Model file for the job. Use its own axes, mm. Give positions to 0.01 mm unless a question says otherwise; leave off trailing zeros. Write each loop counter-clockwise with the first axis right and the second up, starting at its lowest first coordinate (ties: lowest second). Pieces come first, ordered by that corner, then holes. Notation, with made-up numbers: (48, -32) - (77, -32) arc R25 cw to (77, 5) - close; hole circle Ø1 at (87.25, -9). An arc over 180 degrees is marked (long way). Use CSV: the item, a comma, the result in double quotes.
from build123d import *

# Parameters (mm, degrees)
BOSS_EXTRUDE1_DEPTH         = 3.175
FILLET1_R                   = 3.175
F_1_4_0_25_DIAMETER_HOLE1_D = 6.35


with BuildPart() as part:
    # Sketch1 → Boss-Extrude1 (new body)
    with BuildSketch(Plane(origin=(0, 0, 0), x_dir=(1, 0, 0), z_dir=(0, 1, 0))):
        Polygon((-634.164473684, 176.797368421), (413.585526316, 75.197368421), (413.585526316, -115.302631579), (-634.164473684, -115.302631579), align=None)
    extrude(amount=BOSS_EXTRUDE1_DEPTH)

    # Fillet1
    fillet1_edges = [part.edges().sort_by_distance(p)[0] for p in [
        (413.585526316, 1.5875, 115.302631579),
        (-634.164473684, 1.5875, 115.302631579),
        (-634.164473684, 1.5875, -176.797368421),
        (413.585526316, 1.5875, -75.197368421),
    ]]
    fillet(fillet1_edges, radius=FILLET1_R)

    # 1/4 (0.25) Diameter Hole1 (through all)
    with Locations(Plane(origin=(0, 3.175, 0), x_dir=(1, 0, 0), z_dir=(0, 1, 0))):
        with Locations((404.060526316, 65.672368421), (404.060526316, -20.052631579), (404.060526316, -105.777631579), (-624.639473684, -105.777631579), (-624.639473684, 27.572368421), (-624.639473684, 160.922368421)):
            Hole(F_1_4_0_25_DIAMETER_HOLE1_D / 2)


solid = part.part
(1) Saw through at A-A, the plane y = 1.1. List the corners of the cut face in (x, z) (3 decimals), then the cut area to 3 significant figures.
Checked values:
outline,"(-634.164, -173.3) arc R3.175 ccw to (-630.683, -176.46) - (410.717, -75.476) arc R3.175 ccw to (413.586, -72.315) - (413.586, 112.128) arc R3.175 ccw to (410.411, 115.303) - (-630.989, 115.303) arc R3.175 ccw to (-634.164, 112.128) - close; hole circle Ø6.35 at (-624.639, -160.922); hole circle Ø6.35 at (-624.639, -27.572); hole circle Ø6.35 at (-624.639, 105.778); hole circle Ø6.35 at (404.061, -65.672); hole circle Ø6.35 at (404.061, 20.053); hole circle Ø6.35 at (404.061, 105.778)"
area,"253,000 mm^2"
(2) Flat gauge pins, fed straight in: P1, Ø8.5, axis at x = -624.64, z = -160.92, coming from the +Y side (3 decimals); P2, Ø4, axis at x = -624.64, z = 105.78, coming from the +Y side. Where does each tip first touch, or does it go through?
Checked values:
P1,"stops at y = 3.175"
P2,"passes through"
(3) Wall check: probe 1 along Z at (x, y) = (326, 2.9); probe 2 along Z at (x, y) = (-332, 1). Give the ranges that are in metal, low to high. Write a range as [from, to].
Checked values:
probe 1,"z = [-83.69, 115.3]"
probe 2,"z = [-147.5, 115.3]"
(4) Saw through at C-C, the plane x = -406. List the corners of the cut face in (y, z) (3 decimals), then the cut area to 3 significant figures.
Checked values:
outline,"(0, -154.672) - (3.175, -154.672) - (3.175, 115.303) - (0, 115.303) - close"
area,"857 mm^2"
(5) Saw through at B-B, the plane x = -537. List the corners of the cut face in (y, z) (3 decimals).
Checked values:
outline,"(0, -167.375) - (3.175, -167.375) - (3.175, 115.303) - (0, 115.303) - close"
